Autodesk Inventor part; units mm, degrees
ref_plane "YZ Plane" through (0, 0, 0) normal (1, 0, 0) x (0, 1, 0)
ref_plane "XZ Plane" through (0, 0, 0) normal (0, 1, 0) x (-1, 0, 0)
ref_plane "XY Plane" through (0, 0, 0) normal (0, 0, 1) x (1, 0, 0)
sketch "Skizze1" plane through (0, 0, 0) normal (1, 0, 0) x (0, 1, 0)
  line L0 (190, 0) -> (144, 0)
  line L1 (144, 0) -> (144, 300)
  line L2 (144, 300) -> (190, 300)
  line L3 (190, 300) -> (190, 280)
  line L4 (190, 0) -> (190, 20)
  line L5 (163.8, 300) -> (190, 300)
  line L6 (0, 0) -> (0, 300)
  line L7 (190, 280) -> (150, 280)
  line L8 (150, 280) -> (150, 20)
  line L9 (150, 20) -> (190, 20)
  dimension "d0" = 46
  dimension "d1" = 300
  dimension "d2" = 46
  dimension "d3" = 20
  dimension "d9" = 300
  dimension "d48" = 40
revolve "Umdrehung1" add sketch "Skizze1" angle 360 about axis through (0, 0, 0) along (0, 0, 1)
sketch "Skizze3" plane through (0, 0, 0) normal (0, 0, -1) x (-1, 0, 0)
  circle A0 centre (175, 0) radius 5.5
  point P0 (0, 0)
hole "Bohrung2" at (-175, 0, 0) direction (0, 0, 1) diameter 11 depth 25 tip angle 118
pattern_circular "Runde Anordnung2" count 18 over 360 about axis through (0, 0, 150) along (0, 0, -1) of "Bohrung2"
sketch "Skizze12" plane through (0, 0, 300) normal (0, 0, 1) x (1, 0, 0)
  point P0 (0, 0)
  point P1 (-175, 0)
  dimension "d51" = 175
hole "Bohrung3" at (-175, 0, 300) direction (0, 0, -1) diameter 11 depth 30 tip angle 118
pattern_circular "Runde Anordnung3" count 18 over 360 about axis through (0, 0, -10) along (0, 0, 1) of "Bohrung3"
properties part number "Reaktor" material "PET-Kunststoff"
Could you check a few things on this model? Use its own coordinates, in mm. A direction names the side the tool comes from. Give positions to 0.01 mm unless a question says otherwise; leave off trailing zeros. Write each loop counter-clockwise with the first axis right and the second up, starting at its lowest first coordinate (ties: lowest second). Pieces come first, ordered by that corner, then holes. Notation, with made-up numbers: (-17, 68.25) -> (-1, 68.25) arc R17 cw to (-1, 91.25) -> close; hole circle Ø10 at (84, 76). An arc over 180 degrees is marked (long way). Answer as CSV lines item,"result". Start each with the question number.
(1) If we section it at A-A, the plane y = 0: Give the number of separate pieces and of enclosed holes in the cut face, and give its area (3 significant figures).
(2) If we section it at C-C, the plane y = 133.5: Write out the boundary of the cut face in (x, z).
(3) If we section it at D-D, the plane x = 175: Write out the boundary of the cut face in (y, z), and give its area (3 significant figures).
(4) Please list where these lines run through material, in increasing order: line 1 (Z direction, x = 135, y = 107); line 2 (X direction, y = 1, z = 271.5); line 3 (Y direction, x = -175, z = 5).
(5) I'm going to push flat-ended pins straight in: pin 1 Ø8 at (y, z) = (113, 235) entering from -X; pin 2 Ø6 at (x, z) = (121, 119) entering from -Y; pin 3 Ø2 at (x, z) = (-12.5, 204) entering from -Y. Where does each tip first touch, or does it pass through?
(6) Which directions (+Z, -Z, +X, -X, +Y, -Y) give clear straight access to the entire face, cutting with the end or side of a thin tool? Please do faces 5 (the face through (-57, 140, 20)), 6 (the face through (35.84, 173.06, 10.14)).
(7) If we section it at B-B, the plane x = 0: Write out the boundary of the cut face in (y, z), and give its area (3 significant figures).
(8) If we mould it in two halves opening along X, with no side actions, what happens to faces 1 (the face through (148.724, -19.527, 148.18)), 2 (the face through (126, -71, 300)), 3 (the face through (169.63, -1.19, 289.86)), 4 (the face through (-35.84, -173.06, 10.14))? For each: +X half, -X half, draft (parallel to the pull), parting line (faces both ways), or undercut.
Answer list:
1,separate pieces,"6"
1,enclosed holes,"0"
1,area,"5,920 mm^2"
2,outline,"(-135.2, 0) -> (-53.98, 0) -> (-53.98, 300) -> (-135.2, 300) -> (-135.2, 280) -> (-68.39, 280) -> (-68.39, 20) -> (-135.2, 20) -> close; (53.98, 0) -> (135.2, 0) -> (135.2, 20) -> (68.39, 20) -> (68.39, 280) -> (135.2, 280) -> (135.2, 300) -> (53.98, 300) -> close"
3,outline,"(-73.99, 0) -> (-5.5, 0) -> (-5.5, 20) -> (-73.99, 20) -> close; (-73.99, 280) -> (-5.5, 280) -> (-5.5, 300) -> (-73.99, 300) -> close; (5.5, 0) -> (73.99, 0) -> (73.99, 20) -> (5.5, 20) -> close; (5.5, 280) -> (73.99, 280) -> (73.99, 300) -> (5.5, 300) -> close"
3,area,"5,480 mm^2"
4,line 1,"0 to 20, 280 to 300"
4,line 2,"-150 to -144, 144 to 150"
4,line 3,"-73.99 to -5.5, 5.5 to 73.99"
5,pin 1,"x = -103.05"
5,pin 2,"y = -92.61"
5,pin 3,"y = -149.56"
6,face 5,"none"
6,face 6,"+Z, -Z"
7,outline,"(-190, 0) -> (-144, 0) -> (-144, 300) -> (-190, 300) -> (-190, 280) -> (-150, 280) -> (-150, 20) -> (-190, 20) -> close; (144, 0) -> (190, 0) -> (190, 20) -> (150, 20) -> (150, 280) -> (190, 280) -> (190, 300) -> (144, 300) -> close"
7,area,"6,800 mm^2"
8,face 1,"parting line"
8,face 2,"draft"
8,face 3,"undercut"
8,face 4,"undercut"
